Source: CAD feature listing. Evaluate the final solid. Frame: model axes, mm. A direction names the side the tool comes from. Round coordinates to 2 decimals unless told otherwise and drop trailing zeros. Loops run counter-clockwise (first coordinate to the right, second up) from the corner with the lowest first, then second, coordinate; pieces in that order, holes last.
Item 1: Access query for faces 4 (the flat face through (-30, 1, 4)), 5 (the flat face through (26, 1, -7)), 6 (the flat face through (-37, 1, -11.2)). Directions: +Z, -Z, +X, -X, +Y, -Y. A direction counts if a zero-diameter tool reaches every point of the face in a straight line with its end or side. Return the directions, or none.
Item 2: Section query B-B on x = -7. Return loops of the section in (y, z).
Item 3: Ray query, L1, parallel to X at y = 17.5, z = 7; L2, parallel to Z at x = 1, y = 24; L3, parallel to X at y = -29, z = 3.25. Return the intervals inside material, ascending.
Item 4: First-contact query: P1, Ø4, axis at y = 12, z = 8.5, coming from the -X side; P2, Ø10, axis at x = 5, y = -16, coming from the +Z side; P3, Ø4, axis at y = 16.5, z = -7.5, coming from the +X side. Flat tips, straight axial feed; report the tip coordinate or a pass-through.
Item 5: Pull-direction query (X, two-part tool) for faces 1 (the flat face through (16, 1, -7)), 2 (the flat face through (-18, 1, -13)), 3 (the flat face through (-30, 1, 0)); classes: released by +X, released by -X, zero draft, split by the parting line, or undercut.
Item 6: Section query A-A on z = -10. Return loops of the section in (x, y), then the cut area to 3 significant figures.
```python
from build123d import *

# Parameters (mm, degrees)
SKETCH001_W            = 70
SKETCH001_H            = 100
PAD_DEPTH              = 4
SKETCH_W               = 2
SKETCH_H               = 30
PAD001_DEPTH           = 50
PAD001_DEPTH_BACK      = 50
LINEARPATTERN_COUNT    = 3
LINEARPATTERN_PITCH    = 8
LINEARPATTERN001_COUNT = 2
LINEARPATTERN001_PITCH = 51
LINEARPATTERN002_COUNT = 2
LINEARPATTERN002_PITCH = 59
SKETCH002_W            = 7
SKETCH002_H            = 1.8
PAD002_DEPTH           = 50
PAD002_DEPTH_BACK      = 50


with BuildPart() as part:
    # Sketch001 → Pad (new body)
    with BuildSketch(Plane.XY):
        Rectangle(SKETCH001_W, SKETCH001_H)
    extrude(amount=PAD_DEPTH)

    # Sketch → Pad001 (join, two sides)
    with BuildSketch(Plane.XZ) as pad001_sk:
        with Locations((-34, 2)):
            Rectangle(SKETCH_W, SKETCH_H)
    pad001 = extrude(amount=PAD001_DEPTH) + extrude(pad001_sk.sketch, amount=-PAD001_DEPTH_BACK)

    # Mirrored: Pad001 across Sketch V_Axis
    add(pad001.mirror(Plane(origin=(0, 0, 0), x_dir=(0, -1, 0), z_dir=(1, 0, 0))))

    # LinearPattern: Pad001 ×3
    with Locations(*[(i * LINEARPATTERN_PITCH, 0, 0) for i in range(1, LINEARPATTERN_COUNT)]):
        add(pad001)

    # LinearPattern001: Pad001 ×2
    with Locations(*[(i * LINEARPATTERN001_PITCH, 0, 0) for i in range(1, LINEARPATTERN001_COUNT)]):
        add(pad001)

    # LinearPattern002: Pad001 ×2
    with Locations(*[(i * LINEARPATTERN002_PITCH, 0, 0) for i in range(1, LINEARPATTERN002_COUNT)]):
        add(pad001)

    # Sketch002 → Pad002 (join, two sides)
    with BuildSketch(Plane.XZ) as pad002_sk:
        with Locations((36.5, -12.1)):
            Rectangle(SKETCH002_W, SKETCH002_H)
    pad002 = extrude(amount=PAD002_DEPTH) + extrude(pad002_sk.sketch, amount=-PAD002_DEPTH_BACK)

    # Mirrored001: Pad002 across Sketch002 V_Axis
    add(pad002.mirror(Plane(origin=(0, 0, 0), x_dir=(0, -1, 0), z_dir=(1, 0, 0))))


solid = part.part
```
Data:
1. face 4: +Z, +Y, -Y
1. face 5: -Z, +Y, -Y
1. face 6: +Z, -X, +Y, -Y
2. outline: (-50, 0) - (50, 0) - (50, 4) - (-50, 4) - close
3. L1: x = -35 to -33, -27 to -25, -19 to -17, 16 to 18, 24 to 26, 33 to 35
3. L2: z = 0 to 4
3. L3: x = -35 to 35
4. P1: stops at x = -35
4. P2: stops at z = 4
4. P3: stops at x = 35
5. face 1: undercut
5. face 2: zero draft
5. face 3: undercut
6. outline: (-35, -50) - (-33, -50) - (-33, 50) - (-35, 50) - close; (-27, -50) - (-25, -50) - (-25, 50) - (-27, 50) - close; (-19, -50) - (-17, -50) - (-17, 50) - (-19, 50) - close; (16, -50) - (18, -50) - (18, 50) - (16, 50) - close; (24, -50) - (26, -50) - (26, 50) - (24, 50) - close; (33, -50) - (35, -50) - (35, 50) - (33, 50) - close
6. area: 1,200 mm2
